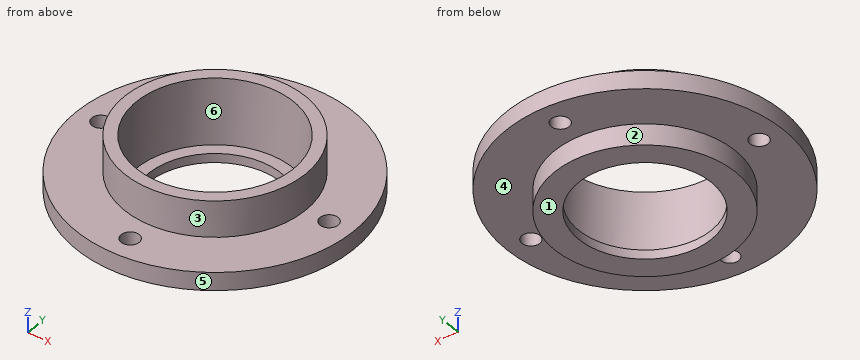
from build123d import *

# Parameters (mm, degrees)
BOSS_EXTRUDE1_DEPTH      = 7.5
BOSS_EXTRUDE1_DEPTH_BACK = 5
SKETCH1_R                = 15
SKETCH1_R_2              = 13
BOSS_EXTRUDE2_DEPTH      = 1.5
BOSS_EXTRUDE2_DEPTH_BACK = 1.5
SKETCH2_R                = 23
SKETCH2_R_2              = 15
SKETCH4_R                = 13
SKETCH4_R_2              = 11
BOSS_EXTRUDE3_DEPTH      = 1.5
SKETCH6_R                = 1.5
CUT_EXTRUDE1_DEPTH       = 10


with BuildPart() as part:
    # Sketch1 → Boss-Extrude1 (new, two sides: drawn at the far end of the back side and taken through both)
    with BuildSketch(Plane.XY.offset(-BOSS_EXTRUDE1_DEPTH_BACK)):
        Circle(SKETCH1_R)
        Circle(SKETCH1_R_2, mode=Mode.SUBTRACT)
    extrude(amount=BOSS_EXTRUDE1_DEPTH + BOSS_EXTRUDE1_DEPTH_BACK)

    # Sketch2 → Boss-Extrude2 (add, two sides: drawn at the far end of the back side and taken through both)
    with BuildSketch(Plane.XY.offset(-BOSS_EXTRUDE2_DEPTH_BACK)):
        Circle(SKETCH2_R)
        Circle(SKETCH2_R_2, mode=Mode.SUBTRACT)
    extrude(amount=BOSS_EXTRUDE2_DEPTH + BOSS_EXTRUDE2_DEPTH_BACK)

    # Sketch4 → Boss-Extrude3 (add)
    with BuildSketch(Plane(origin=(0, 0, -5), x_dir=(-1, 0, 0), z_dir=(0, 0, -1))):
        with Locations(Location((0, 0, 0), (0, 0, 180))):
            Circle(SKETCH4_R)
        Circle(SKETCH4_R_2, mode=Mode.SUBTRACT)
    extrude(amount=-BOSS_EXTRUDE3_DEPTH)

    # Sketch6 → Cut-Extrude1 (cut)
    with BuildSketch(Plane.XY.offset(1.5)):
        with Locations((0, 19)):
            Circle(SKETCH6_R)
        with Locations((19, 0)):
            Circle(SKETCH6_R)
        with Locations((0, -19)):
            Circle(SKETCH6_R)
        with Locations((-19, 0)):
            Circle(SKETCH6_R)
    extrude(amount=-CUT_EXTRUDE1_DEPTH, mode=Mode.SUBTRACT)


solid = part.part
The listing builds one solid part. Answer for the finished solid, in the listing's coordinates (mm). Face numbers are marked on the shaded views. A direction names the side the tool comes from. Round coordinates to 2 decimals unless told otherwise and drop trailing zeros. Write each loop counter-clockwise with the first axis right and the second up, starting at its lowest first coordinate (ties: lowest second). Pieces come first, ordered by that corner, then holes. Notation, with made-up numbers: (74.5, 62.25) - (120.5, 62.25) arc R23 ccw to (120.5, 91.25) - close; hole circle Ø1 at (35, 26). An arc over 180 degrees is marked (long way). Use one line per item in the form item = value. Start each with the question number.
Item 1: A cutting plane is placed at D-D (x = -19). Write down the section's boundary in (y, z), plus the area to 3 significant figures.
Item 2: Find the intervals of material crossed by line 1 (Y direction, x = 0, z = 0); line 2 (Y direction, x = 0, z = -4.5); line 3 (Z direction, x = -11, y = -2), in increasing order. Write a range as [from, to].
Item 3: A cutting plane is placed at A-A (x = 0). Write down the section's boundary in (y, z).
Item 4: A tool of negligible diameter and unlimited length cuts with its end or side. For the marked faces 1, 2 and 3, from which of +Z, -Z, +X, -X, +Y, -Y can it reach the whole face along a straight path? Write none if from no direction.
Item 5: Flat-ended cylindrical pins translate along their axes: pin 1 Ø2.5 at (x, y) = (0, -19) entering from -Z; pin 2 Ø5 at (x, z) = (-7, 0) entering from +Y; pin 3 Ø2 at (y, z) = (12.5, 3) entering from -X; pin 4 Ø3.5 at (x, y) = (0, 19) entering from +Z. Find the tip coordinate at first contact, or state that the pin passes through.
Item 6: A cutting plane is placed at C-C (z = -0.25). Write down the section's boundary in (x, y).
Item 7: Determine the mould class of the marked faces 4, 5 and 6 for opening direction X: +X half, -X half, draft (parallel to the pull), parting line (faces both ways), or undercut.
The answers:
q1.outline = (-12.96, -1.5) - (-1.5, -1.5) - (-1.5, 1.5) - (-12.96, 1.5) - close; (1.5, -1.5) - (12.96, -1.5) - (12.96, 1.5) - (1.5, 1.5) - close
q1.area = 68.8 mm^2
q2.line_1 = [-23, -20.5], [-17.5, -13], [13, 17.5], [20.5, 23]
q2.line_2 = [-15, -11], [11, 15]
q2.line_3 = [-5, -3.5]
q3.outline = (-23, -1.5) - (-20.5, -1.5) - (-20.5, 1.5) - (-23, 1.5) - close; (-17.5, -1.5) - (-15, -1.5) - (-15, -5) - (-11, -5) - (-11, -3.5) - (-13, -3.5) - (-13, 7.5) - (-15, 7.5) - (-15, 1.5) - (-17.5, 1.5) - close; (11, -5) - (15, -5) - (15, -1.5) - (17.5, -1.5) - (17.5, 1.5) - (15, 1.5) - (15, 7.5) - (13, 7.5) - (13, -3.5) - (11, -3.5) - close; (20.5, -1.5) - (23, -1.5) - (23, 1.5) - (20.5, 1.5) - close
q4.face_1 = -Z, +X, -X, +Y, -Y
q4.face_2 = -Z
q4.face_3 = +Z
q5.pin_1 = through
q5.pin_2 = 22.56
q5.pin_3 = -9.63
q5.pin_4 = 1.5
q6.outline = circle Ø46 at (0, 0); hole circle Ø3 at (-19, 0); hole circle Ø26 at (0, 0); hole circle Ø3 at (0, -19); hole circle Ø3 at (0, 19); hole circle Ø3 at (19, 0)
q7.face_4 = draft
q7.face_5 = parting line
q7.face_6 = undercut
